from build123d import *

# Parameters (mm, degrees)
PAD004_DEPTH   = 12.5
THICKNESS002_T = -1
FILLET006_R    = 2
FILLET007_R    = 2


with BuildPart() as part:
    # Sketch009 → Pad004 (new body)
    with BuildSketch(Plane.XY):
        with BuildLine():
            ThreePointArc((-83, 72.5), (-99.5, 56), (-83, 39.5))
            Line((-83, 39.5), (-50.5, 39.5))
            ThreePointArc((-50.5, 39.5), (-34, 56), (-50.5, 72.5))
            Line((-50.5, 72.5), (-83, 72.5))
        make_face()
    extrude(amount=PAD004_DEPTH)

    # Thickness002
    thickness002_openings = [part.faces().sort_by_distance(p)[0] for p in [
        (-66.75, 56, 12.5),
    ]]
    offset(amount=THICKNESS002_T, openings=thickness002_openings)

    # Fillet006
    fillet006_edges = [part.edges().sort_by_distance(p)[0] for p in [
        (-98.5, 56, 1),
        (-66.75, 40.5, 1),
        (-35, 56, 1),
        (-66.75, 71.5, 1),
    ]]
    fillet(fillet006_edges, radius=FILLET006_R)

    # Fillet007
    fillet007_edges = [part.edges().sort_by_distance(p)[0] for p in [
        (-99.5, 56, 0),
        (-66.75, 39.5, 0),
        (-34, 56, 0),
        (-66.75, 72.5, 0),
    ]]
    fillet(fillet007_edges, radius=FILLET007_R)


with BuildPart() as part_1:
    # Body004 placement: moved
    add(part.part.moved(Location((101, -59, 52))))


solid = part_1.part
Verification items for the finished model (mm, model axes). A direction names the side the tool comes from. Coordinates: 2 decimals unless noted, no trailing zeros. Loops run counter-clockwise (first coordinate to the right, second up) from the corner with the lowest first, then second, coordinate; pieces in that order, holes last. Notation, with made-up numbers: M 89.25,-22 L 148.25,-22 A14 cw 148.25,-6 Z; hole C -24.5,69 d11. An arc over 180 degrees is marked long. One line per item, written item: value.
1. Set-up check for faces 4 (the flat face through (34, -3, 52)), 5 (the flat face through (34, 12.5, 60)): record each of +Z, -Z, +X, -X, +Y, -Y from which the full face is reachable in a straight line by a thin tool's end or side.
Answers follow:
face 4: -Z, +X, -X, +Y, -Y
face 5: +Z
2. Gauge pin test, flat ends, axial feed: P1, Ø1, axis at x = 17.5, y = -12.5, coming from the +Z side; P2, Ø3, axis at x = 59, z = 55, coming from the +Y side; P3, Ø1, axis at x = 12.5, z = 57, coming from the -Y side. Record the tip position at first contact, or that the pin passes through.
Answers follow:
P1: z = 53
P2: y = 11.94
P3: y = -18.72
3. Mould release check, pull along Y, two halves, no side actions. Record for faces 1 (the cylindrical face through (34.48, 11.93, 53.6)), 2 (the cylindrical face through (34.02, 12.93, 52.6)), 3 (the flat face through (34, -19.5, 59)): pulls with the +Y half, pulls with the -Y half, needs draft (parallel to the pull), parting line crosses it, or undercut.
Answers follow:
face 1: undercut
face 2: pulls with the +Y half
face 3: pulls with the -Y half
4. Material ranges on line 1 along X through (y, z) = (-3, 57); line 2 along Y through (x, z) = (26, 58.5); line 3 along Z through (x, y) = (55, -11.5), recorded low to high. Write a range as from..to.
Answers follow:
line 1: 1.5..2.5, 66..67
line 2: -19.5..-18.5, 12.5..13.5
line 3: 52..53
5. Section check C-C on y = -3. Record the cut outline in (x, z), plus the area to 3 significant figures.
Answers follow:
outline: M 1.5,54 A2 ccw 3.5,52 L 65,52 A2 ccw 67,54 L 67,64.5 L 66,64.5 L 66,55 A2 cw 64,53 L 4.5,53 A2 cw 2.5,55 L 2.5,64.5 L 1.5,64.5 Z
area: 88.5 mm^2
6. Section check A-A on z = 56. Record the cut outline in (x, y), plus the area to 3 significant figures.
Answers follow:
outline: M 18,-19.5 L 50.5,-19.5 A16.5 ccw 50.5,13.5 L 18,13.5 A16.5 ccw Z; hole M 18,-18.5 L 50.5,-18.5 A15.5 ccw 50.5,12.5 L 18,12.5 A15.5 ccw Z
area: 166 mm^2
7. Section check B-B on x = 36. Record the cut outline in (y, z).
Answers follow:
outline: M -19.5,54 A2 ccw -17.5,52 L 11.5,52 A2 ccw 13.5,54 L 13.5,64.5 L 12.5,64.5 L 12.5,55 A2 cw 10.5,53 L -16.5,53 A2 cw -18.5,55 L -18.5,64.5 L -19.5,64.5 Z
